Part print with two shaded views. Sizes in mm from the minimum x, y, z corner. A direction names the side the tool comes from. Give positions to 0.01 mm unless a question says otherwise; leave off trailing zeros. Write each loop counter-clockwise with the first axis right and the second up, starting at its lowest first coordinate (ties: lowest second). Pieces come first, ordered by that corner, then holes. Notation, with made-up numbers: (40.5, 87) -> (98.5, 87) arc R24 cw to (98.5, 105) -> close; hole circle Ø9 at (-15.75, 83.5). An arc over 180 degrees is marked (long way). Write item = value, one per line. Start each with the question number.
Q1. Mould opens along X. For the marked faces 1, 2, 3 and 4 say: pulls with the +X half, pulls with the -X half, needs draft (parallel to the pull), parting line crosses it, or undercut.
Q2. Saw through at D-D, the plane x = 17. List the corners of the cut face in (y, z).
Q3. Saw through at B-B, the plane x = 10. List the corners of the cut face in (y, z), then the cut area to 3 significant figures.
Q4. Wall check: line 1 (X direction, y = 0.45, z = 10); line 2 (X direction, y = 1.55, z = 10); line 3 (X direction, y = 3.55, z = 10). Give the ranges that are in metal, low to high.
Q5. Saw through at A-A, the plane z = 10. List the corners of the cut face in (x, y), then the cut area to 3 significant figures.
Q6. Tool access for the marked faces 5 and 6: list every direction of +Z, -Z, +X, -X, +Y, -Y with a clear straight run to the whole face (end or side of a thin tool).
Q7. Saw through at C-C, the plane z = 17. List the corners of the cut face in (x, y).
Q8. Drop flat-ended pins along their axis: P1, Ø3.5, axis at x = 10, z = 17, coming from the -Y side; P2, Ø1.5, axis at x = 2, y = 1.5, coming from the -Z side; P3, Ø6, axis at x = 3.5, z = 3, coming from the +Y side; P4, Ø2.5, axis at x = 10, z = 10, coming from the -Y side. Give the stop position or say it passes through.
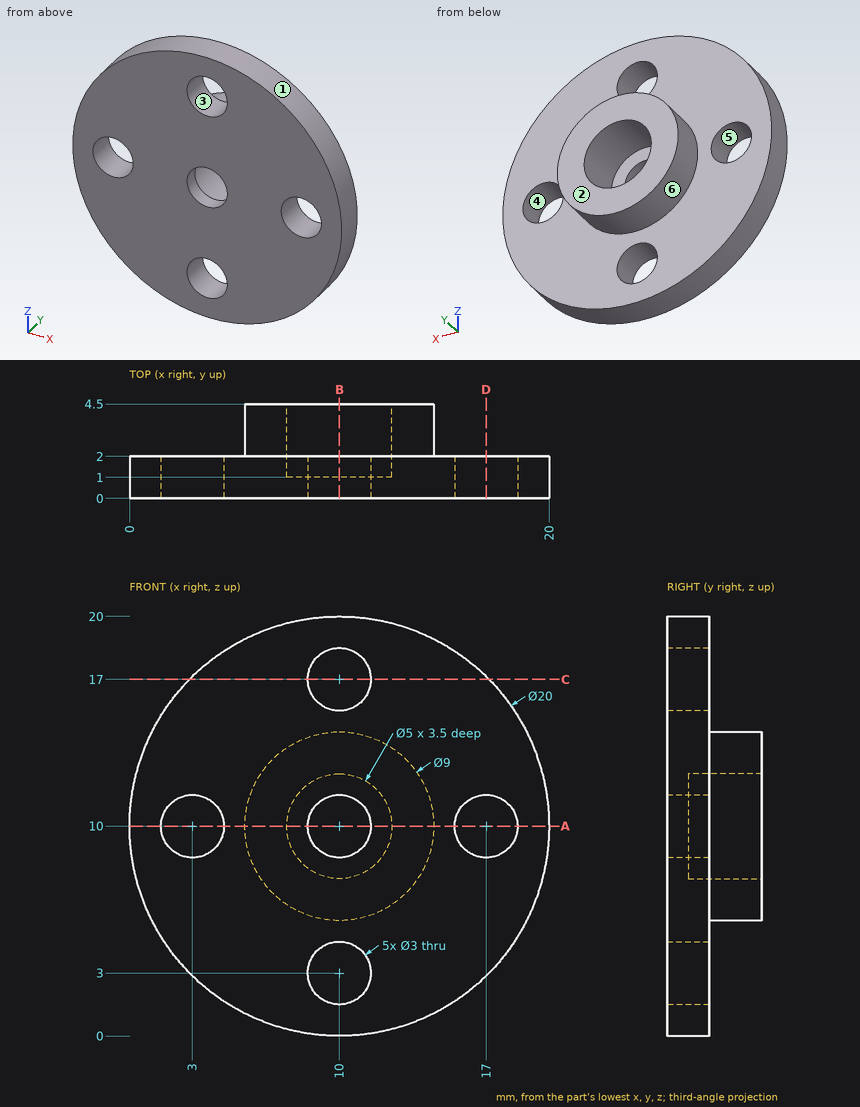
Report:
q1.face_1 = parting line crosses it
q1.face_2 = needs draft
q1.face_3 = undercut
q1.face_4 = undercut
q2.outline = (0, 2.86) -> (2, 2.86) -> (2, 8.5) -> (0, 8.5) -> close; (0, 11.5) -> (2, 11.5) -> (2, 17.14) -> (0, 17.14) -> close
q3.outline = (0, 0) -> (2, 0) -> (2, 1.5) -> (0, 1.5) -> close; (0, 4.5) -> (2, 4.5) -> (2, 5.5) -> (4.5, 5.5) -> (4.5, 7.5) -> (1, 7.5) -> (1, 8.5) -> (0, 8.5) -> close; (0, 11.5) -> (1, 11.5) -> (1, 12.5) -> (4.5, 12.5) -> (4.5, 14.5) -> (2, 14.5) -> (2, 15.5) -> (0, 15.5) -> close; (0, 18.5) -> (2, 18.5) -> (2, 20) -> (0, 20) -> close
q3.area = 30.0 mm2
q4.line_1 = 0 to 1.5, 4.5 to 8.5, 11.5 to 15.5, 18.5 to 20
q4.line_2 = 0 to 1.5, 4.5 to 7.5, 12.5 to 15.5, 18.5 to 20
q4.line_3 = 5.5 to 7.5, 12.5 to 14.5
q5.outline = (0, 0) -> (1.5, 0) -> (1.5, 2) -> (0, 2) -> close; (4.5, 0) -> (8.5, 0) -> (8.5, 1) -> (7.5, 1) -> (7.5, 4.5) -> (5.5, 4.5) -> (5.5, 2) -> (4.5, 2) -> close; (11.5, 0) -> (15.5, 0) -> (15.5, 2) -> (14.5, 2) -> (14.5, 4.5) -> (12.5, 4.5) -> (12.5, 1) -> (11.5, 1) -> close; (18.5, 0) -> (20, 0) -> (20, 2) -> (18.5, 2) -> close
q5.area = 30.0 mm2
q6.face_5 = +Y, -Y
q6.face_6 = +Y
q7.outline = (2.86, 0) -> (8.5, 0) -> (8.5, 2) -> (2.86, 2) -> close; (11.5, 0) -> (17.14, 0) -> (17.14, 2) -> (11.5, 2) -> close
q8.P1 = 0
q8.P2 = 3.11
q8.P3 = 2
q8.P4 = through
